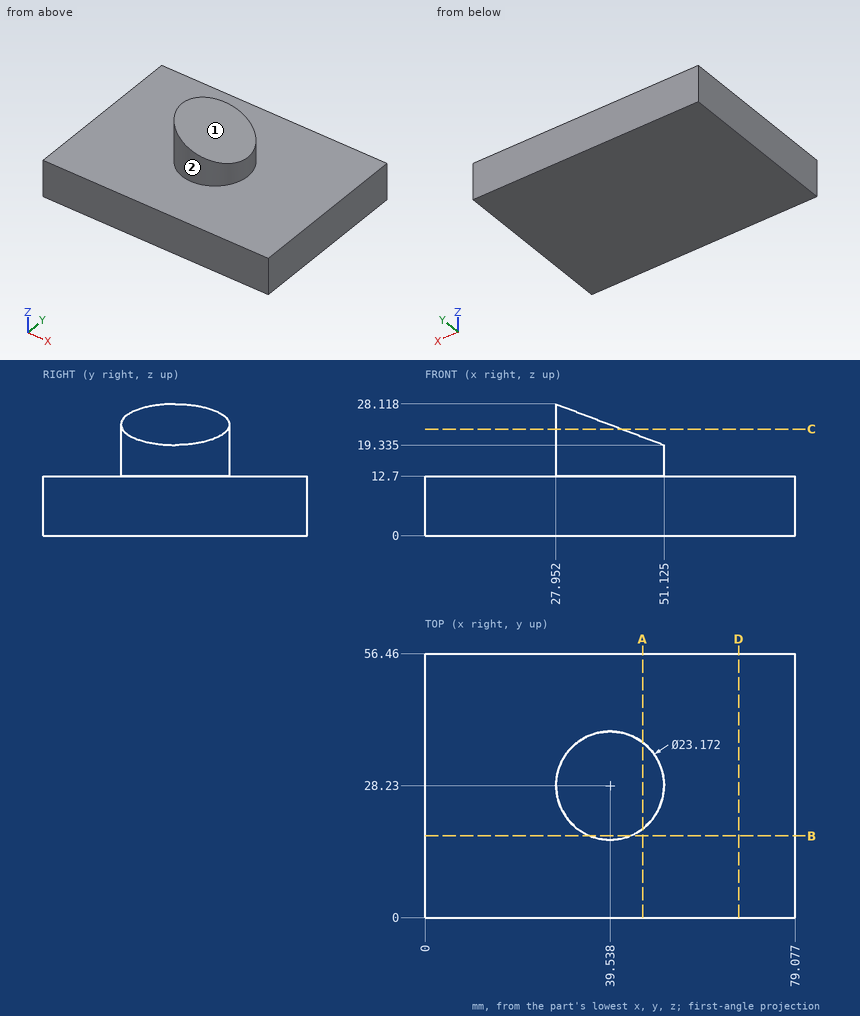
Drawing for the job (mm, zero at the part's lowest x, y, z). A direction names the side the tool comes from. Round coordinates to 2 decimals unless told otherwise and drop trailing zeros. Write each loop counter-clockwise with the first axis right and the second up, starting at its lowest first coordinate (ties: lowest second). Pieces come first, ordered by that corner, then holes. Notation, with made-up numbers: M 11,-1.5 L 43,-1.5 A5 cw 43,7.5 Z; hole C 28.25,65 d10. An arc over 180 degrees is marked long. One line per question, with ' | ' between items.
1. Pin check, flat tips, straight feed: pin 1 Ø2 at (x, y) = (33.5, 50) entering from +Z; pin 2 Ø8 at (y, z) = (30, 22.5) entering from -X; pin 3 Ø5 at (y, z) = (47, 11.5) entering from -X; pin 4 Ø8 at (x, y) = (35.5, 24) entering from +Z. Stop position of each tip, or through.
Working result:
pin 1: z = 12.7 | pin 2: x = 27.95 | pin 3: x = 0 | pin 4: z = 26.77
2. Cut at D-D on x = 67. Write the cut outline in (y, z).
Working result:
outline: M 0,0 L 56.46,0 L 56.46,12.7 L 0,12.7 Z
3. Cut at C-C on z = 22.75. Write the cut outline in (x, y), and give its area (3 significant figures).
Working result:
outline: M 42.11,16.93 L 42.11,39.53 A11.59 ccw long Z | area: 270 mm2
4. Cut at A-A on x = 46.5. Write the cut outline in (y, z).
Working result:
outline: M 0,0 L 56.46,0 L 56.46,12.7 L 37.49,12.7 L 37.49,21.09 L 18.97,21.09 L 18.97,12.7 L 0,12.7 Z
5. Which spindle directions (+Z, -Z, +X, -X, +Y, -Y) get a long thin tool onto all of the face, cutting with end or side? Do the marked faces 1 and 2. Say none if no direction does.
Working result:
face 1: +Z, +X, +Y, -Y | face 2: +Z
6. Probe L1, parallel to Z at x = 46, y = 50; L2, parallel to Y at x = 38, z = 19.75; L3, parallel to Z at x = 34.5, y = 18 (1 decimal). List the from-to ranges inside material, lowest first. Write a range as from..to.
Working result:
L1: 0..12.7 | L2: 16.75..39.71 | L3: 0..25.6
7. Cut at B-B on y = 17.5. Write the cut outline in (x, z).
Working result:
outline: M 0,0 L 79.08,0 L 79.08,12.7 L 43.91,12.7 L 43.91,22.07 L 35.17,25.38 L 35.17,12.7 L 0,12.7 Z
